```python
from build123d import *

# Parameters (mm, degrees)
F0_W     = 47.9552
F0_H     = 7.874
F1_DEPTH = 3.175
F2_W     = 44.704
F2_H     = 4.7498
F2_R     = 1.4224
F3_DEPTH = 2.0828
F2_R_2   = 0.8255
F4_DEPTH = 2.0828
F5_W     = 49.073476
F5_H     = 9.354642
F5_W_2   = 46.99
F5_H_2   = 7.0866
F6_DEPTH = 0.508


with BuildPart() as f1:
    # F0 (on Top) → F1 (new body)
    with BuildSketch(Plane.XY):
        Rectangle(F0_W, F0_H)
    extrude(amount=F1_DEPTH)

    # F2 (on face) → F3 (cut)
    with BuildSketch(Plane.XY.offset(3.175)):
        Rectangle(F2_W, F2_H)
        with Locations((-16.002, 0)):
            Circle(F2_R, mode=Mode.SUBTRACT)
        with Locations((-8.001, 0)):
            Circle(F2_R, mode=Mode.SUBTRACT)
        Circle(F2_R, mode=Mode.SUBTRACT)
        with Locations((8.001, 0)):
            Circle(F2_R, mode=Mode.SUBTRACT)
        with Locations((16.002, 0)):
            Circle(F2_R, mode=Mode.SUBTRACT)
    extrude(amount=-F3_DEPTH, mode=Mode.SUBTRACT)

    # F2 (on face) → F4 (cut)
    with BuildSketch(Plane.XY.offset(3.175)):
        with Locations((16.002, 0)):
            Circle(F2_R_2)
        with Locations((8.001, 0)):
            Circle(F2_R_2)
        with Locations((-8.001, 0)):
            Circle(F2_R_2)
        Circle(F2_R_2)
        with Locations((-16.002, 0)):
            Circle(F2_R_2)
    extrude(amount=-F4_DEPTH, mode=Mode.SUBTRACT)

    # F5 (on face) → F6 (cut)
    with BuildSketch(Plane.XY.offset(3.175)):
        Rectangle(F5_W, F5_H)
        Rectangle(F5_W_2, F5_H_2, mode=Mode.SUBTRACT)
    extrude(amount=-F6_DEPTH, mode=Mode.SUBTRACT)


solid = f1.part
```
For this review, take the finished solid that the model builds, in its own axes (mm). A direction names the side the tool comes from. Coordinates: 2 decimals unless noted, no trailing zeros. Write each loop counter-clockwise with the first axis right and the second up, starting at its lowest first coordinate (ties: lowest second). Pieces come first, ordered by that corner, then holes.
(1) Add section C-C on x = -18. Give the boundary of the cut face in (y, z) (3 decimals).
(2) For pin 1 Ø0.8 at (x, y) = (0, 0) entering from +Z; pin 2 Ø2.5 at (x, y) = (0, 0) entering from +Z (3 decimals), all flat-tipped, find the tip position at first contact; note any pin that passes through.
(3) Tool access review of faces 1 (the face through (0, 2, 1.092)), 2 (the face through (-15, 0, 3.175)): name each direction out of +Z, -Z, +X, -X, +Y, -Y from which nothing blocks a thin tool from reaching the whole face with its end or side.
(4) Wall thickness on probe 1 along Y at (x, z) = (0, 2.3); probe 2 along Y at (x, z) = (9.5, 2.5); probe 3 along Y at (x, z) = (0, 2.7): over which ranges is each line inside the solid? List them lowest first.
(5) Add section A-A on z = 1.5. Count the separate pieces of the cut face and the enclosed holes in it, then the cut area to 3 significant figures.
(6) The part is to be moulded in two halves that separate along Y. For faces 3 (the face through (0, 2.375, 2)), 4 (the face through (0, -3.937, 1)), 5 (the face through (9, 0, 3.175)), say which applies: +Y half, -Y half, draft (parallel to the pull), parting line (faces both ways), or undercut.
Answer sheet:
1. outline: (-3.937, 0) - (3.937, 0) - (3.937, 2.667) - (3.543, 2.667) - (3.543, 3.175) - (2.375, 3.175) - (2.375, 1.092) - (-2.375, 1.092) - (-2.375, 3.175) - (-3.543, 3.175) - (-3.543, 2.667) - (-3.937, 2.667) - close
2. pin 1: stops at z = 1.09
2. pin 2: stops at z = 3.175
3. face 1: +Z
3. face 2: +Z, +X, -X, +Y, -Y
4. probe 1: y = -3.94 to -2.37, -1.42 to -0.83, 0.83 to 1.42, 2.37 to 3.94
4. probe 2: y = -3.94 to -2.37, 2.37 to 3.94
4. probe 3: y = -3.54 to -2.37, -1.42 to -0.83, 0.83 to 1.42, 2.37 to 3.54
5. separate pieces: 6
5. enclosed holes: 6
5. area: 186 mm2
6. face 3: undercut
6. face 4: -Y half
6. face 5: draft
